```python
from build123d import *

# Parameters (mm, degrees)
SKETCH1_W           = 400
SKETCH1_H           = 70
BOSS_EXTRUDE1_DEPTH = 12
SKETCH3_W           = 60
SKETCH3_H           = 55
CUT_EXTRUDE1_DEPTH  = 8
SKETCH4_R           = 1.5
CUT_EXTRUDE2_DEPTH  = 401
SKETCH5_W           = 60
SKETCH5_H           = 3
BOSS_EXTRUDE2_DEPTH = 10


with BuildPart() as part:
    # Sketch1 → Boss-Extrude1 (new body)
    with BuildSketch(Plane.XY):
        Rectangle(SKETCH1_W, SKETCH1_H)
    extrude(amount=BOSS_EXTRUDE1_DEPTH)

    # Sketch3 → Cut-Extrude1 (cut)
    with BuildSketch(Plane.XY.offset(12)):
        with Locations((-90, 2)):
            Rectangle(SKETCH3_W, SKETCH3_H)
        with Locations((90, 2)):
            Rectangle(SKETCH3_W, SKETCH3_H)
    extrude(amount=-CUT_EXTRUDE1_DEPTH, mode=Mode.SUBTRACT)

    # Sketch4 → Cut-Extrude2 (cut, through all)
    with BuildSketch(Plane.ZY.offset(200)):
        with Locations((8, 25)):
            Circle(SKETCH4_R)
    extrude(amount=-CUT_EXTRUDE2_DEPTH, mode=Mode.SUBTRACT)

    # Sketch5 → Boss-Extrude2 (add)
    with BuildSketch(Plane.XY.offset(12)):
        with Locations((-90, 31)):
            Rectangle(SKETCH5_W, SKETCH5_H)
        with Locations((90, 31)):
            Rectangle(SKETCH5_W, SKETCH5_H)
    extrude(amount=BOSS_EXTRUDE2_DEPTH)


solid = part.part
```
Model file for the job. Use its own axes, mm. A direction names the side the tool comes from. Coordinates: 2 decimals unless noted, no trailing zeros. Loops run counter-clockwise (first coordinate to the right, second up) from the corner with the lowest first, then second, coordinate; pieces in that order, holes last. Notation, with made-up numbers: (-21, 67.25) - (1, 67.25) arc R26 cw to (1, 105.25) - close; hole circle Ø2 at (-13, 42.25). An arc over 180 degrees is marked (long way). Answer as a JSON object with one key per item and string values. Group by question number.
(1) Cut at C-C (x = 77.5). Give the cut face in (y, z), then the cut area to 3 significant figures.
(2) Cut at A-A (x = 4). Give the cut face in (y, z).
(3) Cut at B-B (z = 17.25). Give the cut face in (x, y), then the cut area to 3 significant figures.
(4) Two-plate mould, pull along Y, no slides. Class faces 1 (the face through (-120, 2, 8)), 2 (the face through (200, 0, 6)), 3 (the face through (90, 32.5, 17)), 4 (the face through (-3, -35, 6)): released by +Y, released by -Y, zero draft, split by the parting line, or undercut.
(5) Tool access for faces 5 (the face through (-200, 0, 6)), 6 (the face through (-90, 29.5, 13)), 7 (the face through (-90, 32.5, 17)): list every direction of +Z, -Z, +X, -X, +Y, -Y with a clear straight run to the whole face (end or side of a thin tool).
(6) Flat gauge pins, fed straight in: pin 1 (16.5 mm diameter, centred on x = 92.5, y = -1, fed in from +Z); pin 2 (0.9 mm diameter, centred on y = 30.5, z = 15, fed in from -X); pin 3 (12 mm diameter, centred on x = 27, y = 3, fed in from -Z); pin 4 (5 mm diameter, centred on x = 19, y = 10, fed in from +Z). Where does each tip first touch, or does it go through?
(7) Probe line 1 along X through (y, z) = (-13, 11); line 2 along Y through (x, z) = (146, 8); line 3 along Y through (x, z) = (103.5, 17.5). List the from-to ranges inside material, lowest first.
Geometry says:
{
 "1": {"outline": "(-35, 0) - (35, 0) - (35, 12) - (32.5, 12) - (32.5, 22) - (29.5, 22) - (29.5, 4) - (-25.5, 4) - (-25.5, 12) - (-35, 12) - close", "area": "430 mm^2"},
 "2": {"outline": "(-35, 0) - (35, 0) - (35, 12) - (-35, 12) - close; hole circle Ø3 at (25, 8)"},
 "3": {"outline": "(-120, 29.5) - (-60, 29.5) - (-60, 32.5) - (-120, 32.5) - close; (60, 29.5) - (120, 29.5) - (120, 32.5) - (60, 32.5) - close", "area": "360 mm^2"},
 "4": {"face 1": "undercut", "face 2": "zero draft", "face 3": "released by +Y", "face 4": "released by -Y"},
 "5": {"face 5": "+Z, -Z, -X, +Y, -Y", "face 6": "+Z", "face 7": "+Z, +X, -X, +Y"},
 "6": {"pin 1": "stops at z = 4", "pin 2": "stops at x = -120", "pin 3": "stops at z = 0", "pin 4": "stops at z = 12"},
 "7": {"line 1": "x = -200 to -120, -60 to 60, 120 to 200", "line 2": "y = -35 to 23.5, 26.5 to 35", "line 3": "y = 29.5 to 32.5"}
}
